Read the model definition and answer for the solid it produces. Units are mm, in the model's axes. Face numbers are marked on the shaded views. A direction names the side the tool comes from. Give positions to 0.01 mm unless a question says otherwise; leave off trailing zeros. Order: outer loops, then holes, each group sorted by start corner. A loop starts at its lowest first (then second) coordinate and runs counter-clockwise, first axis right, second up. Notation, with made-up numbers: (1, -19.75) -> (46, -19.75) arc R24 ccw to (46, 17.25) -> close; hole circle Ø3 at (-24, -22). An arc over 180 degrees is marked (long way). Use one line per item in the form item = value.
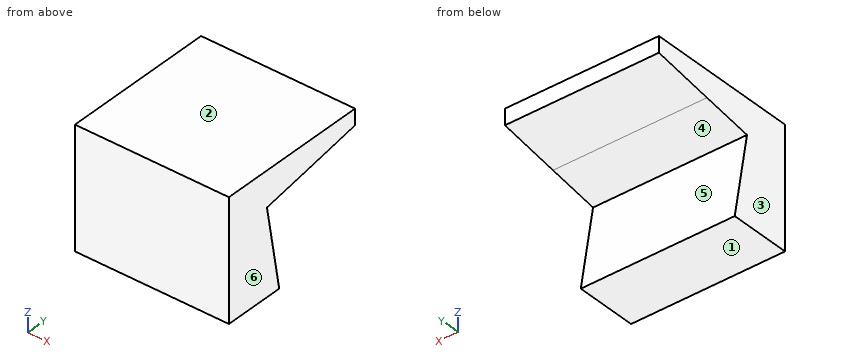
```python
from build123d import *

# Parameters (mm, degrees)
SKETCH1_W           = 78
SKETCH1_H           = 78
BOSS_EXTRUDE1_DEPTH = 78
CUT_EXTRUDE2_DEPTH  = 118
SKETCH3_W           = 78
SKETCH3_H           = 17.233329778
CUT_EXTRUDE3_DEPTH  = 96.269447677


with BuildPart() as part:
    # Sketch1 → Boss-Extrude1 (new body)
    with BuildSketch(Plane(origin=(0, 0, 0), x_dir=(1, 0, 0), z_dir=(0, 1, 0))):
        Rectangle(SKETCH1_W, SKETCH1_H)
    extrude(amount=BOSS_EXTRUDE1_DEPTH)

    # Sketch2 → Cut-Extrude2 (cut, through all)
    with BuildSketch(Plane(origin=(39, 0, 0), x_dir=(0, 0, -1), z_dir=(1, 0, 0))):
        Polygon((-21.767253197, 0.141749363), (-21.767253197, 78), (-39, 78), (-39, 0), align=None)
        Polygon((-4.012108483, 23.522620279), (39, 31.106815501), (39, 78), (-13.767253197, 78), (-8.378409218, 48.285142253), align=None)
    extrude(amount=-CUT_EXTRUDE2_DEPTH, mode=Mode.SUBTRACT)

    # Sketch3 → Cut-Extrude3 (cut, through all)
    with BuildSketch(Plane(origin=(0, 0.320775974, 0.002638569), x_dir=(1, 0, 0), z_dir=(0, 0.9999661716212329, 0.00822530322693927))):
        with Locations((0, -30.382015804)):
            Rectangle(SKETCH3_W, SKETCH3_H)
    extrude(amount=-CUT_EXTRUDE3_DEPTH, mode=Mode.SUBTRACT)


solid = part.part
```
Item 1: The part is cut by section B-B on z = -33.5. Give the vertices of the cut face in (x, y), and give its area (3 significant figures).
Checks:
outline = (-39, 0) -> (39, 0) -> (39, 30.14) -> (-39, 30.14) -> close
area = 2,350 mm²
Item 2: Given pin 1 Ø1 at (x, z) = (5, -20.5) entering from +Y; pin 2 Ø12 at (x, z) = (-16, -6) entering from +Y; pin 3 Ø4 at (x, z) = (-5, -7) entering from +Y, each flat-ended and moving along its own axis, determine where each tip first touches the part or whether it passes through.
Checks:
pin_1 = 27.93
pin_2 = 26.35
pin_3 = 25.82
Item 3: Straight lines are drawn through the part: L1, parallel to Z at x = -3.5, y = 55.5; L2, parallel to Y at x = -17, z = -1; L3, parallel to Z at x = -1, y = 47.5. For each, find the intervals that lie inside material, in ascending order. Write a range as from..to.
Checks:
L1 = 9.69..21.77
L2 = 0..24.41
L3 = 8.24..21.77
Item 4: The part is cut by section A-A on x = 22. Give the vertices of the cut face in (y, z).
Checks:
outline = (0, -39) -> (31.11, -39) -> (23.52, 4.01) -> (48.29, 8.38) -> (78, 13.77) -> (78, 21.77) -> (0.14, 21.77) -> (0, 21.77) -> close
Item 5: Determine the mould class of the marked faces 1, 2, 3 and 4 for opening direction Z: +Z half, -Z half, draft (parallel to the pull), parting line (faces both ways), or undercut.
Checks:
face_1 = -Z half
face_2 = +Z half
face_3 = draft
face_4 = undercut
Item 6: The part is cut by section C-C on y = 61. Give the vertices of the cut face in (x, z).
Checks:
outline = (-39, 10.68) -> (39, 10.68) -> (39, 21.77) -> (-39, 21.77) -> close
Item 7: Which of the six approach directions +Z, -Z, +X, -X, +Y, -Y give full straight-line access (tool end or side, diameter ignored) to the marked faces 5 and 6?
Checks:
face_5 = +X, -X, +Y
face_6 = +Z, -Z, +X, +Y, -Y
